Geometry: final body of the model. Coordinates: model frame, mm. Face numbers are marked on the shaded views. Give positions to 0.01 mm unless a question says otherwise; leave off trailing zeros. Loops run counter-clockwise (first coordinate to the right, second up) from the corner with the lowest first, then second, coordinate; pieces in that order, holes last. Notation, with made-up numbers: (66, 17.25) - (107, 17.25) arc R19 ccw to (107, 24.25) - close; hole circle Ø4 at (77, 32.5). An arc over 180 degrees is marked (long way). Use CSV: the item, a comma, the result in double quotes. Start each with the question number.
```python
from build123d import *

# Parameters (mm, degrees)
SKETCH1_R                = 19.939
BOSS_EXTRUDE1_DEPTH      = 91.44
BOSS_EXTRUDE2_DEPTH      = 20.32
BOSS_EXTRUDE2_DEPTH_BACK = 20.32
SKETCH3_R                = 16.51
SKETCH4_R                = 16.51
CUT_EXTRUDE1_DEPTH       = 102.880441814
CUT_EXTRUDE2_REACH       = 113.277
CUT_EXTRUDE2_END_RADIUS  = 16.51
SKETCH5_R                = 13.335


with BuildPart() as part:
    # Sketch1 → Boss-Extrude1 (new body)
    with BuildSketch(Plane.XY):
        Circle(SKETCH1_R)
    extrude(amount=BOSS_EXTRUDE1_DEPTH)

    # Sketch3 → Boss-Extrude2 (add, two sides: drawn at the far end of the back side and taken through both)
    with BuildSketch(Plane(origin=(0, 19.939, 0), x_dir=(1, 0, 0), z_dir=(0, 1, 0)).offset(-BOSS_EXTRUDE2_DEPTH_BACK)):
        with Locations(Location((0, -45.72, 0), (0, 0, 270))):
            Circle(SKETCH3_R)
    extrude(amount=BOSS_EXTRUDE2_DEPTH + BOSS_EXTRUDE2_DEPTH_BACK)

    # Sketch4 → Cut-Extrude1 (cut, through all)
    with BuildSketch(Plane.XY.offset(91.44)):
        Circle(SKETCH4_R)
    extrude(amount=-CUT_EXTRUDE1_DEPTH, mode=Mode.SUBTRACT)

    # Cut-Extrude2: up to this cylinder (the profile starts outside it)
    cut_extrude2_end = Plane(origin=(0, 0, 45.72), z_dir=(0, 0, 1)) * Cylinder(CUT_EXTRUDE2_END_RADIUS, 260.574, mode=Mode.PRIVATE)
    # Sketch5 → Cut-Extrude2 (cut, up to the surface)
    with BuildSketch(Plane(origin=(0, 40.259, 0), x_dir=(1, 0, 0), z_dir=(0, 1, 0)), mode=Mode.PRIVATE) as cut_extrude2_sk1:
        with Locations(Location((0, -45.72, 0), (0, 0, 270))):
            Circle(SKETCH5_R)
    cut_extrude2_tool1 = extrude(cut_extrude2_sk1.sketch, amount=-CUT_EXTRUDE2_REACH, mode=Mode.PRIVATE) - cut_extrude2_end
    add(cut_extrude2_tool1.solids().sort_by_distance((0, 40.259, 45.72))[0], mode=Mode.SUBTRACT)


solid = part.part
```
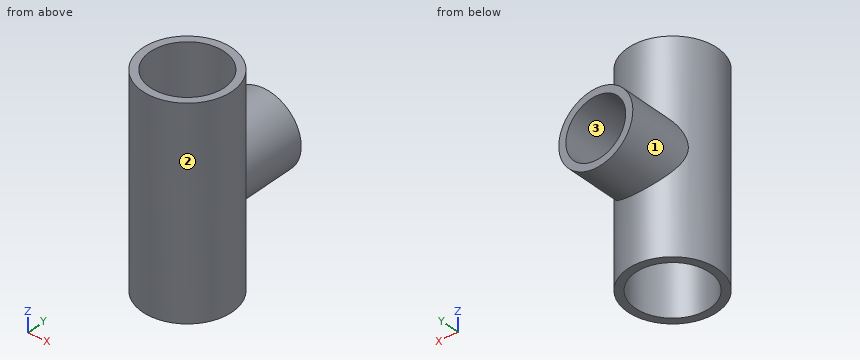
Item 1: Section D-D (z = 45.72). Output: boundary loops of the cut face in (x, y) (3 decimals).
Item 2: Ray query, probe 1 along Y at (x, z) = (0, 29); probe 2 along X at (y, z) = (-15, 48); probe 3 along Y at (x, z) = (13, 11). Return the intervals inside material, ascending.
Item 3: Section B-B (x = -1). Output: boundary loops of the cut face in (y, z).
Item 4: Mould query, pull axis Z, two halves, no side actions, for the marked faces 1, 2 and 3. Classes: pulls with the +Z half, pulls with the -Z half, needs draft (parallel to the pull), parting line crosses it, or undercut.
Item 5: Pin query (flat end, axial travel): pin 1 Ø5 at (x, y) = (12.5, 3.5) entering from +Z; pin 2 Ø4 at (y, z) = (28.5, 55) entering from +X; pin 3 Ø2 at (y, z) = (6, 60.5) entering from -X; pin 4 Ø1 at (y, z) = (18, 11) entering from +X. Return the tip coordinate at first contact, or that it passes through.
Item 6: Section A-A (y = 0). Output: boundary loops of the cut face in (x, z).
Item 7: Section C-C (y = 18.5). Output: boundary loops of the cut face in (x, z) (3 decimals).
Outcome:
1,outline,"(-16.51, 11.18) arc R19.939 ccw (long way) to (16.51, 11.18) - (16.51, 40.259) - (13.335, 40.259) - (13.335, 9.734) arc R16.51 cw (long way) to (-13.335, 9.734) - (-13.335, 40.259) - (-16.51, 40.259) - close"
2,probe 1,"y = -19.94 to -16.51, 16.51 to 19.94"
2,probe 2,"x = -13.14 to -6.9, 6.9 to 13.14"
2,probe 3,"y = -15.12 to -10.18, 10.18 to 15.12"
3,outline,"(-19.91, 0) - (-16.48, 0) - (-16.48, 91.44) - (-19.91, 91.44) - close; (16.48, 0) - (19.91, 0) - (19.91, 29.24) - (40.26, 29.24) - (40.26, 32.42) - (16.48, 32.42) - close; (16.48, 59.02) - (40.26, 59.02) - (40.26, 62.2) - (19.91, 62.2) - (19.91, 91.44) - (16.48, 91.44) - close"
4,face 1,"parting line crosses it"
4,face 2,"needs draft"
4,face 3,"undercut"
5,pin 1,"passes through"
5,pin 2,"stops at x = 14.82"
5,pin 3,"stops at x = -19.3"
5,pin 4,"stops at x = 9.56"
6,outline,"(-19.94, 0) - (-16.51, 0) - (-16.51, 91.44) - (-19.94, 91.44) - close; (16.51, 0) - (19.94, 0) - (19.94, 91.44) - (16.51, 91.44) - close"
7,outline,"(-7.437, 0) - (7.437, 0) - (7.437, 30.98) arc R16.51 ccw to (7.437, 60.46) - (7.437, 91.44) - (-7.437, 91.44) - (-7.437, 60.46) arc R16.51 ccw to (-7.437, 30.98) - close; hole circle Ø26.67 at (0, 45.72)"
